Work out the finished part from the listing and answer in its coordinate system (mm). A direction names the side the tool comes from. Coordinates: 2 decimals unless noted, no trailing zeros. Write each loop counter-clockwise with the first axis right and the second up, starting at its lowest first coordinate (ties: lowest second). Pieces come first, ordered by that corner, then holes. Notation, with made-up numbers: M -11,-15 L 38,-15 A23 ccw 38,4 Z; hole C 83.5,14.25 d11. An arc over 180 degrees is marked long. Use CSV: the item, a comma, the result in double quotes.
Autodesk Inventor part; units mm, degrees
ref_plane "YZ Plane" through (0, 0, 0) normal (1, 0, 0) x (0, 1, 0)
ref_plane "XZ Plane" through (0, 0, 0) normal (0, 1, 0) x (-1, 0, 0)
ref_plane "XY Plane" through (0, 0, 0) normal (0, 0, 1) x (1, 0, 0)
sketch "Sketch1" plane through (0, 0, 0) normal (0, 1, 0) x (-1, 0, 0)
  line L0 (-17.5, -17.5) -> (17.5, -17.5)
  line L1 (17.5, -17.5) -> (17.5, 17.5)
  line L2 (17.5, 17.5) -> (-17.5, 17.5)
  line L3 (-17.5, 17.5) -> (-17.5, -17.5)
  line L4 (-17.5, -17.5) -> (17.5, 17.5) construction
  line L5 (17.5, -17.5) -> (-17.5, 17.5) construction
  point P0 (0, 0)
  dimension "d0" = 35
extrude "Extrusion1" add sketch "Sketch1" along normal blind 4
sketch "Sketch2" plane through (0, 0, 0) normal (0, 1, 0) x (1, 0, 0)
  circle A0 centre (0, 0) radius 16
  dimension "d3" = 32
extrude "Extrusion2" add sketch "Sketch2" along normal blind 36.8
sketch "Sketch3" plane through (0, 36.8, 0) normal (0, 1, 0) x (1, 0, 0)
  circle A0 centre (0, 0) radius 9.5
  dimension "d6" = 19
extrude "Extrusion3" add sketch "Sketch3" along normal blind 2
sketch "Sketch4" plane through (0, 36.8, 0) normal (0, 1, 0) x (1, 0, 0)
  circle A0 centre (0, 0) radius 3
  dimension "d9" = 6
extrude "Extrusion4" add sketch "Sketch4" along normal blind 18
sketch "Sketch5" plane through (0, 36.8, 0) normal (0, 1, 0) x (1, 0, 0)
  line L0 (24.5, 0) -> (-24.5, 0)
  line L1 (0, 24.5) -> (0, -24.5)
  point P0 (13, 0)
  dimension "d49" = 13
hole "Hole1" at (13, 36.8, 0) direction (0, -1, 0) diameter 2.459 depth 8.8 tip angle 118
pattern_circular "Circular Pattern1" count 4 over 360 about axis through (0, -10, 0) along (0, 1, 0) of "Hole1"
chamfer "Chamfer1" distance 3 angle 45 4 edges at (17.5, 2, -17.5) (-17.5, 2, -17.5) (17.5, 2, 17.5) (-17.5, 2, 17.5)
sketch "Sketch7" plane through (0, 0, 0) normal (0, 1, 0) x (-1, 0, 0)
  circle A0 centre (0, 0) radius 11
  dimension "d30" = 22
extrude "Extrusion5" cut sketch "Sketch7" along normal blind 2
sketch "Sketch8" plane through (0, 0, 0) normal (0, 1, 0) x (-1, 0, 0)
  line L0 (13, 13) -> (-13, 13)
  line L1 (-13, 13) -> (-13, -13)
  line L2 (-13, -13) -> (13, -13)
  line L3 (13, -13) -> (13, 13)
  line L4 (13, 13) -> (-13, -13) construction
  line L5 (-13, 13) -> (13, -13) construction
  point P0 (0, 0)
  dimension "d33" = 26
hole "Hole3" at (13, 0, 13) at (-13, 0, 13) at (-13, 0, -13) at (13, 0, -13) direction (0, 1, 0) diameter 3.5 depth 4
sketch "Sketch9" plane through (0, 4, 0) normal (0, 1, 0) x (1, 0, 0)
  circle A0 centre (-13, -13) radius 1.75
  circle A1 centre (-13, 13) radius 1.75
  circle A2 centre (13, 13) radius 1.75
  circle A3 centre (13, -13) radius 1.75
  point P0 (0, 0)
  point P1 (-13.6978, -15.9176)
  point P2 (-15.9176, -13.6978)
  point P3 (13.6978, 15.9176)
  point P4 (15.9176, 13.6978)
  point P5 (14.7912, 17.2088)
  point P6 (-14.7912, -17.2088)
  point P7 (-17.2088, -14.7912)
  point P8 (17.2088, 14.7912)
hole "Hole4" at (-13, 4, 13) at (-13, 4, -13) at (13, 4, -13) at (13, 4, 13) direction (0, -1, 0) diameter 6.6 depth 3 tip angle 118
sketch "Sketch10" plane through (0, 54.8, 0) normal (0, 1, 0) x (1, 0, 0)
  line L0 (-4.6716, -4.4668) -> (-2, -4.4668)
  line L1 (-2, -4.4668) -> (-2, 4.6167)
  line L2 (-2, 4.6167) -> (-4.6716, 4.6167)
  line L3 (-4.6716, 4.6167) -> (-4.6716, -4.4668)
  point P0 (0, 0)
  dimension "d53" = 2
extrude "Extrusion6" cut sketch "Sketch10" against normal blind 12
properties part number "911-42-reducer-long"
Item 1: The part is cut by section A-A (y = 31). Write down the section's boundary in (x, z), then the cut area to 3 significant figures.
Answer:
outline,"C 0,0 d32; hole C -13,0 d2.46; hole C 0,-13 d2.46; hole C 0,13 d2.46; hole C 13,0 d2.46"
area,"785 mm2"
Item 2: The part is cut by section C-C (x = -4). Write down the section's boundary in (y, z), then the cut area to 3 significant figures.
Answer:
outline,"M 0,-17.5 L 4,-17.5 L 4,-15.49 L 36.8,-15.49 L 36.8,-8.62 L 38.8,-8.62 L 38.8,8.62 L 36.8,8.62 L 36.8,15.49 L 4,15.49 L 4,17.5 L 0,17.5 L 0,10.25 L 2,10.25 L 2,-10.25 L 0,-10.25 Z"
area,"1,150 mm2"
Item 3: Given pin 1 (8 mm diameter, centred on x = -0.5, y = 46.5, fed in from +Z); pin 2 (4 mm diameter, centred on y = 35, z = 9, fed in from -X); pin 3 (2 mm diameter, centred on y = 49.5, z = 0, fed in from -X); pin 4 (3 mm diameter, centred on x = 13, z = -13, fed in from +Y), each flat-ended and moving along its own axis, determine where each tip first touches the part or whether it passes through.
Answer:
pin 1,"stops at z = 3"
pin 2,"stops at x = -14.39"
pin 3,"stops at x = -2"
pin 4,"passes through"
Item 4: A tool of negligible diameter and unlimited length cuts with its end or side. For faces 1 (the face through (-16, 2, 16)), 2 (the face through (11.78, 32.34, -0.16)), 3 (the face through (2.38, 0.99, 10.74)), 4 (the face through (-10.992, 2.479, 10.381)), from which of +Z, -Z, +X, -X, +Y, -Y can it reach the whole face along a straight path? Write none if from no direction.
Answer:
face 1,"+Z, -X, +Y, -Y"
face 2,"+Y"
face 3,"-Y"
face 4,"none"
Item 5: The part is cut by section B-B (z = -5). Write down the section's boundary in (x, y), then the cut area to 3 significant figures.
Answer:
outline,"M -17.5,0 L -9.8,0 L -9.8,2 L 9.8,2 L 9.8,0 L 17.5,0 L 17.5,4 L 15.2,4 L 15.2,36.8 L 8.08,36.8 L 8.08,38.8 L -8.08,38.8 L -8.08,36.8 L -15.2,36.8 L -15.2,4 L -17.5,4 Z"
area,"1,130 mm2"
Item 6: Consider probe 1 along Z at (x, y) = (13, 0.05); probe 2 along Z at (x, y) = (0, 31.5); probe 3 along X at (y, z) = (2.05, 13). Determine where each line is inside the solid, lowest interval first.
Answer:
probe 1,"z = -17.5 to -14.75, -11.25 to 11.25, 14.75 to 17.5"
probe 2,"z = -16 to -14.23, -11.77 to 11.77, 14.23 to 16"
probe 3,"x = -17.5 to -16.3, -9.7 to 9.7, 16.3 to 17.5"
Item 7: For a pull along X with two mould halves and no side action, classify faces 5 (the face through (15.008, 2.479, 10.381)), 6 (the face through (17.5, 2, 0)), 7 (the face through (2.86, 46.69, 0.9)), 8 (the face through (0, 54.8, 0)) as released by +X, released by -X, zero draft, split by the parting line, or undercut.
Answer:
face 5,"undercut"
face 6,"released by +X"
face 7,"split by the parting line"
face 8,"zero draft"
Item 8: The part is cut by section D-D (y = 25). Write down the section's boundary in (x, z).
Answer:
outline,"C 0,0 d32"
